from build123d import *

# Parameters (mm, degrees)
SKETCH1_W               = 25.4
SKETCH1_H               = 50.8
BOSS_EXTRUDE1_DEPTH     = 453.936862
SKETCH2_W               = 19.05
SKETCH2_H               = 48.768
CUT_EXTRUDE1_DEPTH      = 458.47620122
CUT_EXTRUDE4_DEPTH      = 458.47620122
CUT_EXTRUDE4_DEPTH_BACK = 458.47620122
SKETCH5_R               = 3.175


with BuildPart() as part:
    # Sketch1 → Boss-Extrude1 (new body)
    with BuildSketch(Plane(origin=(0, 0, 0), x_dir=(0, 0, -1), z_dir=(1, 0, 0))):
        with Locations((12.7, 25.4)):
            Rectangle(SKETCH1_W, SKETCH1_H)
    extrude(amount=BOSS_EXTRUDE1_DEPTH)

    # Sketch2 → Cut-Extrude1 (cut, through all)
    with BuildSketch(Plane(origin=(453.936862, 0, 0), x_dir=(0, 0, -1), z_dir=(1, 0, 0))):
        with Locations((12.7, 25.4)):
            Rectangle(SKETCH2_W, SKETCH2_H)
    extrude(amount=-CUT_EXTRUDE1_DEPTH, mode=Mode.SUBTRACT)

    # Sketch5 → Cut-Extrude4 (cut, two sides: drawn at the far end of the back side and taken through both)
    with BuildSketch(Plane.XY.offset(-CUT_EXTRUDE4_DEPTH_BACK)):
        with Locations((12.7, 38.1)):
            Circle(SKETCH5_R)
        with Locations((38.1, 38.1)):
            Circle(SKETCH5_R)
        with Locations((12.7, 12.7)):
            Circle(SKETCH5_R)
        with Locations((38.1, 12.7)):
            Circle(SKETCH5_R)
        with Locations((63.5, 38.1)):
            Circle(SKETCH5_R)
        with Locations((63.5, 12.7)):
            Circle(SKETCH5_R)
        with Locations((441.236862, 38.1)):
            Circle(SKETCH5_R)
        with Locations((441.236862, 12.7)):
            Circle(SKETCH5_R)
        with Locations((415.836862, 38.1)):
            Circle(SKETCH5_R)
        with Locations((415.836862, 12.7)):
            Circle(SKETCH5_R)
    extrude(amount=CUT_EXTRUDE4_DEPTH + CUT_EXTRUDE4_DEPTH_BACK, mode=Mode.SUBTRACT)


solid = part.part
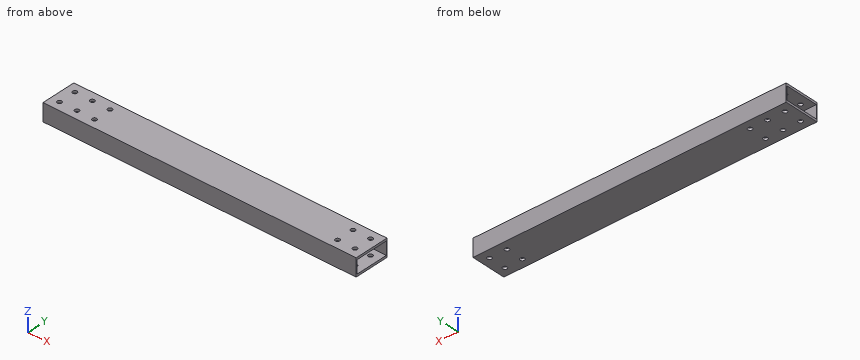
Geometry check sheet. Reference: the model listing, model coordinates, mm. Give positions to 0.01 mm unless a question says otherwise; leave off trailing zeros. Write each loop counter-clockwise with the first axis right and the second up, starting at its lowest first coordinate (ties: lowest second). Pieces come first, ordered by that corner, then holes. Notation, with made-up numbers: (26.25, 89.5) - (79.25, 89.5) arc R18 ccw to (79.25, 121.5) - close; hole circle Ø9 at (-6, 5.5). An arc over 180 degrees is marked (long way). Put each result on its own line as item: value.
1. Sectioned sample at B-B, the plane z = -14. Enter the section's corners in (x, y), plus the area to 3 significant figures.
Ans:
outline: (0, 0) - (453.94, 0) - (453.94, 1.02) - (0, 1.02) - close; (0, 49.78) - (453.94, 49.78) - (453.94, 50.8) - (0, 50.8) - close
area: 922 mm²
2. Go/stop test with flat-tipped pins: pin 1 (8.5 mm diameter, centred on x = 441.24, y = 12.7, fed in from -Z); pin 2 (4 mm diameter, centred on x = 12.7, y = 12.7, fed in from -Z). Record where each tip stops, or that it passes through.
Ans:
pin 1: stops at z = -25.4
pin 2: passes through
3. Thickness scan on line 1 (Y direction, x = 12.7, z = -23) (3 decimals); line 2 (X direction, y = 12.7, z = -24.4) (3 decimals); line 3 (Z direction, x = 247, y = 24.5) (3 decimals). Record the ranges inside material, lowest first.
Ans:
line 1: y = 0 to 9.525, 15.875 to 34.925, 41.275 to 50.8
line 2: x = 0 to 9.525, 15.875 to 34.925, 41.275 to 60.325, 66.675 to 412.662, 419.012 to 438.062, 444.412 to 453.937
line 3: z = -25.4 to -22.225, -3.175 to 0
4. Sectioned sample at A-A, the plane y = 23. Enter the section's corners in (x, z) (3 decimals), plus the area to 3 significant figures.
Ans:
outline: (0, -25.4) - (453.937, -25.4) - (453.937, -22.225) - (0, -22.225) - close; (0, -3.175) - (453.937, -3.175) - (453.937, 0) - (0, 0) - close
area: 2,880 mm²
5. Sectioned sample at C-C, the plane x = 192.5. Enter the section's corners in (y, z) (3 decimals), plus the area to 3 significant figures.
Ans:
outline: (0, -25.4) - (50.8, -25.4) - (50.8, 0) - (0, 0) - close; hole (1.016, -22.225) - (49.784, -22.225) - (49.784, -3.175) - (1.016, -3.175) - close
area: 361 mm²
